The listing builds one solid part. Answer for the finished solid, in the listing's coordinates (mm). Face numbers are marked on the shaded views. A direction names the side the tool comes from. Coordinates: 2 decimals unless noted, no trailing zeros. Order: outer loops, then holes, each group sorted by start corner. A loop starts at its lowest first (then second) coordinate and runs counter-clockwise, first axis right, second up. Notation, with made-up numbers: (32.25, 84.5) -> (71.25, 84.5) arc R10 cw to (71.25, 99.5) -> close; hole circle Ø2 at (58, 84.5). An arc over 180 degrees is marked (long way). Put each result on its own line as item: value. Start each with the question number.
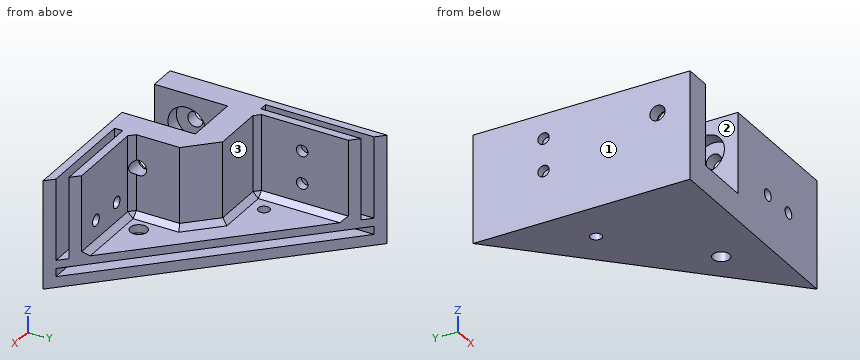
```python
from build123d import *

# Parameters (mm, degrees)
DODANIE_WYCI_GNI_CIE1_DEPTH     = 4
DODANIE_WYCI_GNI_CIE2_DEPTH     = 3
DODANIE_WYCI_GNI_CIE3_DEPTH     = 3
DODANIE_WYCI_GNI_CIE4_DEPTH     = 30
WYTNIJ_WYCI_GNI_CIE1_DEPTH      = 15.5
WYTNIJ_WYCI_GNI_CIE1_DEPTH_BACK = 15.5
SZKIC5_R                        = 7
SZKIC6_R                        = 2.802594562
WYTNIJ_WYCI_GNI_CIE2_DEPTH      = 121
SFAZOWANIE1_SIZE                = 2
SZKIC7_R                        = 3.1
SZKIC7_R_2                      = 2.1
WYTNIJ_WYCI_GNI_CIE3_DEPTH      = 118.046999107
SZKIC8_R                        = 2.1
WYTNIJ_WYCI_GNI_CIE4_DEPTH      = 115.197197864
SZKIC9_R                        = 2.1
WYTNIJ_WYCI_GNI_CIE5_DEPTH      = 115.197197864


with BuildPart() as part:
    # Szkic1 → Dodanie-wyciągnięcie1 (new body)
    with BuildSketch(Plane.XY):
        Polygon((0, 0), (80, 0), (0, 80), align=None)
    extrude(amount=DODANIE_WYCI_GNI_CIE1_DEPTH)

    # Szkic2 → Dodanie-wyciągnięcie2 (add)
    with BuildSketch(Plane.XY.offset(4)):
        Polygon((3, 77), (3, 3), (77, 3), (80, 0), (0, 0), (0, 80), align=None)
    extrude(amount=DODANIE_WYCI_GNI_CIE2_DEPTH)

    # Szkic3 → Dodanie-wyciągnięcie3 (add)
    with BuildSketch(Plane.XY.offset(7)):
        Polygon((80, 0), (77, 3), (3, 77), (0, 80), (0, 0), align=None)
    extrude(amount=DODANIE_WYCI_GNI_CIE3_DEPTH)

    # Szkic4 → Dodanie-wyciągnięcie4 (add)
    with BuildSketch(Plane.XY.offset(10)):
        Polygon((30.2, 0), (80, 0), (77, 3), (40, 3), (40, 6), (74, 6), (71, 9), (40, 9), (40, 27), (30, 37), (9, 37), (9, 71), (6, 74), (6, 37), (3, 37), (3, 77), (0, 80), (0, 0), (9.8, 0), (9.8, 27), (30.2, 27), align=None)
    extrude(amount=DODANIE_WYCI_GNI_CIE4_DEPTH)

    # Szkic5 → Wytnij-wyciągnięcie1 (cut, two sides: drawn at the far end of the back side and taken through both)
    with BuildSketch(Plane(origin=(20, 0, 0), x_dir=(0, 0, -1), z_dir=(1, 0, 0)).offset(-WYTNIJ_WYCI_GNI_CIE1_DEPTH_BACK)):
        with Locations((-28, 12)):
            Circle(SZKIC5_R)
    extrude(amount=WYTNIJ_WYCI_GNI_CIE1_DEPTH + WYTNIJ_WYCI_GNI_CIE1_DEPTH_BACK, mode=Mode.SUBTRACT)

    # Szkic6 → Wytnij-wyciągnięcie2 (cut, through all)
    with BuildSketch(Plane.ZY):
        with Locations((28, 12)):
            Circle(SZKIC6_R)
    extrude(amount=-WYTNIJ_WYCI_GNI_CIE2_DEPTH, mode=Mode.SUBTRACT)

    # Sfazowanie1
    # the kernel refuses this chamfer: 2 mm, written as the material it adds along each edge
    with BuildSketch(Plane(origin=(10.333333333, 38.333333333, 11.333333333), x_dir=(-0.7071067811865475, 0.7071067811865475, 0), z_dir=(-0.5773502691896258, -0.5773502691896258, -0.5773502691896258))) as sfazowanie1_piece_1_section:
        Polygon((-1.414213562, -0.816496581), (1.414213562, -0.816496581), (0, 1.632993162), align=None)
    sfazowanie1_piece_1 = extrude(amount=2.540341184, mode=Mode.PRIVATE)
    sfazowanie1_piece_1 = split(sfazowanie1_piece_1, bisect_by=Plane(origin=(9, 37, 10), z_dir=(0, 1, 0)), keep=Keep.TOP, mode=Mode.PRIVATE)
    sfazowanie1_piece_1 = split(sfazowanie1_piece_1, bisect_by=Plane(origin=(9, 37, 10), z_dir=(1, 0, 0)), keep=Keep.TOP, mode=Mode.PRIVATE)
    sfazowanie1_piece_1 = split(sfazowanie1_piece_1, bisect_by=Plane(origin=(9, 37, 10), z_dir=(0, 0, 1)), keep=Keep.TOP, mode=Mode.PRIVATE)
    add(sfazowanie1_piece_1)
    with BuildSketch(Plane(origin=(41.333333333, 10.333333333, 11.333333333), x_dir=(0, -0.7071067811865475, 0.7071067811865475), z_dir=(-0.5773502691896258, -0.5773502691896258, -0.5773502691896258))) as sfazowanie1_piece_2_section:
        Polygon((-1.414213562, -0.816496581), (1.414213562, -0.816496581), (0, 1.632993162), align=None)
    sfazowanie1_piece_2 = extrude(amount=2.540341184, mode=Mode.PRIVATE)
    sfazowanie1_piece_2 = split(sfazowanie1_piece_2, bisect_by=Plane(origin=(40, 9, 10), z_dir=(0, 0, 1)), keep=Keep.TOP, mode=Mode.PRIVATE)
    sfazowanie1_piece_2 = split(sfazowanie1_piece_2, bisect_by=Plane(origin=(40, 9, 10), z_dir=(0, 1, 0)), keep=Keep.TOP, mode=Mode.PRIVATE)
    sfazowanie1_piece_2 = split(sfazowanie1_piece_2, bisect_by=Plane(origin=(40, 9, 10), z_dir=(1, 0, 0)), keep=Keep.TOP, mode=Mode.PRIVATE)
    add(sfazowanie1_piece_2)
    with BuildSketch(Plane(origin=(9, 37, 4.856634024), x_dir=(1, 0, 0), z_dir=(0, 0, 1))) as sfazowanie1_piece_3_section:
        Polygon((SFAZOWANIE1_SIZE, 0), (0, SFAZOWANIE1_SIZE), (0, 0), align=None)
    sfazowanie1_piece_3 = extrude(amount=35.143365976, mode=Mode.PRIVATE)
    sfazowanie1_piece_3 = split(sfazowanie1_piece_3, bisect_by=Plane(origin=(9, 37, 7), z_dir=(0, 0, 1)), keep=Keep.TOP, mode=Mode.PRIVATE)
    add(sfazowanie1_piece_3)
    with BuildSketch(Plane(origin=(76.143365976, 9, 10), x_dir=(0, 0, 1), z_dir=(-1, 0, 0))) as sfazowanie1_piece_4_section:
        Polygon((SFAZOWANIE1_SIZE, 0), (0, SFAZOWANIE1_SIZE), (0, 0), align=None)
    sfazowanie1_piece_4 = extrude(amount=41.286731952, mode=Mode.PRIVATE)
    sfazowanie1_piece_4 = split(sfazowanie1_piece_4, bisect_by=Plane(origin=(73.571682988, 6.428317012, 10), z_dir=(-0.7071067811865476, -0.7071067811865476, 0)), keep=Keep.TOP, mode=Mode.PRIVATE)
    add(sfazowanie1_piece_4)
    with BuildSketch(Plane(origin=(40, 9, 10), x_dir=(0, 0, 1), z_dir=(0, 1, 0))) as sfazowanie1_piece_5_section:
        Polygon((SFAZOWANIE1_SIZE, 0), (0, SFAZOWANIE1_SIZE), (0, 0), align=None)
    sfazowanie1_piece_5 = extrude(amount=23.143365976, mode=Mode.PRIVATE)
    sfazowanie1_piece_5 = split(sfazowanie1_piece_5, bisect_by=Plane(origin=(49, 18, 10), z_dir=(-0.7071067811865482, -0.7071067811865468, 0)), keep=Keep.TOP, mode=Mode.PRIVATE)
    add(sfazowanie1_piece_5)
    with BuildSketch(Plane(origin=(40, 9, 4.856634024), x_dir=(1, 0, 0), z_dir=(0, 0, 1))) as sfazowanie1_piece_6_section:
        Polygon((SFAZOWANIE1_SIZE, 0), (0, SFAZOWANIE1_SIZE), (0, 0), align=None)
    sfazowanie1_piece_6 = extrude(amount=35.143365976, mode=Mode.PRIVATE)
    sfazowanie1_piece_6 = split(sfazowanie1_piece_6, bisect_by=Plane(origin=(40, 9, 7), z_dir=(0, 0, 1)), keep=Keep.TOP, mode=Mode.PRIVATE)
    sfazowanie1_piece_6 = sfazowanie1_piece_6 - Plane(origin=(40, 12, 28), x_dir=(0, 0, 1), z_dir=(-1, 0, 0)) * Cylinder(2.802594562, 79, mode=Mode.PRIVATE)
    add(sfazowanie1_piece_6)
    with BuildSketch(Plane(origin=(43.63690896, 23.36309104, 10), x_dir=(0, 0, 1), z_dir=(-0.7071067811865468, 0.7071067811865482, 0))) as sfazowanie1_piece_7_section:
        Polygon((SFAZOWANIE1_SIZE, 0), (0, SFAZOWANIE1_SIZE), (0, 0), align=None)
    sfazowanie1_piece_7 = extrude(amount=24.428867576, mode=Mode.PRIVATE)
    sfazowanie1_piece_7 = split(sfazowanie1_piece_7, bisect_by=Plane(origin=(40, 23.36309104, 10), z_dir=(-1, 0, 0)), keep=Keep.TOP, mode=Mode.PRIVATE)
    sfazowanie1_piece_7 = split(sfazowanie1_piece_7, bisect_by=Plane(origin=(43.63690896, 37, 10), z_dir=(0, -1, 0)), keep=Keep.TOP, mode=Mode.PRIVATE)
    add(sfazowanie1_piece_7)
    with BuildSketch(Plane(origin=(9, 31.856634024, 10), x_dir=(0, 0, 1), z_dir=(0, 1, 0))) as sfazowanie1_piece_8_section:
        Polygon((SFAZOWANIE1_SIZE, 0), (0, SFAZOWANIE1_SIZE), (0, 0), align=None)
    sfazowanie1_piece_8 = extrude(amount=44.286731952, mode=Mode.PRIVATE)
    sfazowanie1_piece_8 = split(sfazowanie1_piece_8, bisect_by=Plane(origin=(28.571682988, 51.428317012, 10), z_dir=(-0.7071067811865476, -0.7071067811865476, 0)), keep=Keep.TOP, mode=Mode.PRIVATE)
    add(sfazowanie1_piece_8)
    with BuildSketch(Plane(origin=(35.143365976, 37, 10), x_dir=(0, 0, 1), z_dir=(-1, 0, 0))) as sfazowanie1_piece_9_section:
        Polygon((SFAZOWANIE1_SIZE, 0), (0, SFAZOWANIE1_SIZE), (0, 0), align=None)
    sfazowanie1_piece_9 = extrude(amount=31.286731952, mode=Mode.PRIVATE)
    sfazowanie1_piece_9 = split(sfazowanie1_piece_9, bisect_by=Plane(origin=(32.571682988, 34.428317012, 10), z_dir=(-0.7071067811865482, -0.7071067811865468, 0)), keep=Keep.TOP, mode=Mode.PRIVATE)
    sfazowanie1_piece_9 = split(sfazowanie1_piece_9, bisect_by=Plane(origin=(6, 37, 10), z_dir=(1, 0, 0)), keep=Keep.TOP, mode=Mode.PRIVATE)
    add(sfazowanie1_piece_9)
    with BuildSketch(Plane(origin=(40, 9, 10), x_dir=(0, 0, 1), z_dir=(0, 1, 0))) as sfazowanie1_piece_10a_section:
        Polygon((SFAZOWANIE1_SIZE, 0), (0, SFAZOWANIE1_SIZE), (0, 0), align=None)
    sfazowanie1_piece_10a = extrude(amount=23.143365976, mode=Mode.PRIVATE)
    sfazowanie1_piece_10a = split(sfazowanie1_piece_10a, bisect_by=Plane(origin=(49, 18, 10), z_dir=(0.7071067811865482, 0.7071067811865468, 0)), keep=Keep.TOP, mode=Mode.PRIVATE)
    with BuildSketch(Plane(origin=(43.63690896, 23.36309104, 10), x_dir=(0, 0, 1), z_dir=(-0.7071067811865468, 0.7071067811865482, 0))) as sfazowanie1_piece_10b_section:
        Polygon((SFAZOWANIE1_SIZE, 0), (0, SFAZOWANIE1_SIZE), (0, 0), align=None)
    sfazowanie1_piece_10b = extrude(amount=24.428867576, mode=Mode.PRIVATE)
    sfazowanie1_piece_10b = split(sfazowanie1_piece_10b, bisect_by=Plane(origin=(40, 23.36309104, 10), z_dir=(1, 0, 0)), keep=Keep.TOP, mode=Mode.PRIVATE)
    sfazowanie1_piece_10 = sfazowanie1_piece_10a & sfazowanie1_piece_10b
    add(sfazowanie1_piece_10)
    with BuildSketch(Plane(origin=(43.63690896, 23.36309104, 10), x_dir=(0, 0, 1), z_dir=(-0.7071067811865468, 0.7071067811865482, 0))) as sfazowanie1_piece_11a_section:
        Polygon((SFAZOWANIE1_SIZE, 0), (0, SFAZOWANIE1_SIZE), (0, 0), align=None)
    sfazowanie1_piece_11a = extrude(amount=24.428867576, mode=Mode.PRIVATE)
    sfazowanie1_piece_11a = split(sfazowanie1_piece_11a, bisect_by=Plane(origin=(43.63690896, 37, 10), z_dir=(0, 1, 0)), keep=Keep.TOP, mode=Mode.PRIVATE)
    with BuildSketch(Plane(origin=(35.143365976, 37, 10), x_dir=(0, 0, 1), z_dir=(-1, 0, 0))) as sfazowanie1_piece_11b_section:
        Polygon((SFAZOWANIE1_SIZE, 0), (0, SFAZOWANIE1_SIZE), (0, 0), align=None)
    sfazowanie1_piece_11b = extrude(amount=26.143365976, mode=Mode.PRIVATE)
    sfazowanie1_piece_11b = split(sfazowanie1_piece_11b, bisect_by=Plane(origin=(32.571682988, 34.428317012, 10), z_dir=(0.7071067811865482, 0.7071067811865468, 0)), keep=Keep.TOP, mode=Mode.PRIVATE)
    sfazowanie1_piece_11 = sfazowanie1_piece_11a & sfazowanie1_piece_11b
    add(sfazowanie1_piece_11)

    # Szkic7 → Wytnij-wyciągnięcie3 (cut, through all)
    with BuildSketch(Plane.XY.offset(10)):
        with Locations((47, 16)):
            Circle(SZKIC7_R)
        with Locations((16, 44)):
            Circle(SZKIC7_R_2)
    extrude(amount=-WYTNIJ_WYCI_GNI_CIE3_DEPTH, mode=Mode.SUBTRACT)

    # Szkic8 → Wytnij-wyciągnięcie4 (cut, through all)
    with BuildSketch(Plane(origin=(0, 9, 0), x_dir=(1, 0, 0), z_dir=(0, 1, 0))):
        with Locations(Location((49, -19, 0), (0, 0, 180))):
            Circle(SZKIC8_R)
        with Locations(Location((62, -19, 0), (0, 0, 180))):
            Circle(SZKIC8_R)
    extrude(amount=-WYTNIJ_WYCI_GNI_CIE4_DEPTH, mode=Mode.SUBTRACT)

    # Szkic9 → Wytnij-wyciągnięcie5 (cut, through all)
    with BuildSketch(Plane(origin=(9, 0, 0), x_dir=(0, 0, -1), z_dir=(1, 0, 0))):
        with Locations((-31, 54)):
            Circle(SZKIC9_R)
        with Locations((-19, 54)):
            Circle(SZKIC9_R)
    extrude(amount=-WYTNIJ_WYCI_GNI_CIE5_DEPTH, mode=Mode.SUBTRACT)


solid = part.part
```
(1) Each of these flat-tipped pins is pushed along its axis until it touches: P1, Ø1, axis at x = 38, z = 28, coming from the +Y side; P2, Ø5, axis at y = 18, z = 32.5, coming from the +X side; P3, Ø5.5, axis at y = 54, z = 19, coming from the +X side. Where does it stop, or does it pass through?
(2) The part is cut by section A-A on x = 62. Determine the outline of the cut face in (y, z).
(3) A tool of negligible diameter and unlimited length cuts with its end or side. For the marked faces 1, 2 and 3, from which of +Z, -Z, +X, -X, +Y, -Y can it reach the whole face along a straight path? Write none if from no direction.
(4) The part is cut by section C-C on z = 8.5. Determine the outline of the cut face in (x, y).
(5) Find the intervals of material crossed by L1, parallel to X at y = 11.5, z = 22.5; L2, parallel to Z at x = 6.55, y = 12; L3, parallel to X at y = 63, z = 30.5, in increasing order.
(6) The part is cut by section D-D on y = 54. Count the separate pieces of the cut face and the enclosed holes in it, plus the area to 3 significant figures.
(7) The part is cut by section B-B on y = 44. Determine the outline of the cut face in (x, z).
Worked out:
1. P1: y = 29.5
1. P2: x = 40
1. P3: x = 9
2. outline: (0, 0) -> (18, 0) -> (18, 4) -> (3, 4) -> (3, 7) -> (18, 7) -> (18, 10) -> (11, 10) -> (9, 12) -> (9, 16.9) -> (6, 16.9) -> (6, 10) -> (3, 10) -> (3, 16.9) -> (0, 16.9) -> close; (0, 21.1) -> (3, 21.1) -> (3, 40) -> (0, 40) -> close; (6, 21.1) -> (9, 21.1) -> (9, 40) -> (6, 40) -> close
3. face 1: +Z, -Z, -X, +Y, -Y
3. face 2: +Z, -Y
3. face 3: +Z, +X, +Y
4. outline: (0, 0) -> (80, 0) -> (0, 80) -> close; hole circle Ø4.2 at (16, 44); hole circle Ø6.2 at (47, 16)
5. L1: 0 to 4.5, 35.5 to 40
5. L2: 0 to 4, 7 to 21, 35 to 40
5. L3: 0 to 3, 6 to 9
6. separate pieces: 5
6. enclosed holes: 0
6. area: 323 mm2
7. outline: (0, 0) -> (13.9, 0) -> (13.9, 4) -> (3, 4) -> (3, 7) -> (13.9, 7) -> (13.9, 10) -> (11, 10) -> (9, 12) -> (9, 40) -> (6, 40) -> (6, 10) -> (3, 10) -> (3, 40) -> (0, 40) -> close; (18.1, 0) -> (36, 0) -> (36, 4) -> (18.1, 4) -> close; (18.1, 7) -> (36, 7) -> (36, 10) -> (18.1, 10) -> close
